Part print with two shaded views. Sizes in mm from the minimum x, y, z corner. Give positions to 0.01 mm unless a question says otherwise; leave off trailing zeros. Write each loop counter-clockwise with the first axis right and the second up, starting at its lowest first coordinate (ties: lowest second). Pieces come first, ordered by that corner, then holes. Notation, with made-up numbers: (59, -22) -> (76, -22) arc R26 cw to (76, 6) -> close; hole circle Ø9 at (83, -26). An arc over 180 degrees is marked (long way). Answer as a JSON object with one key per item and string values.
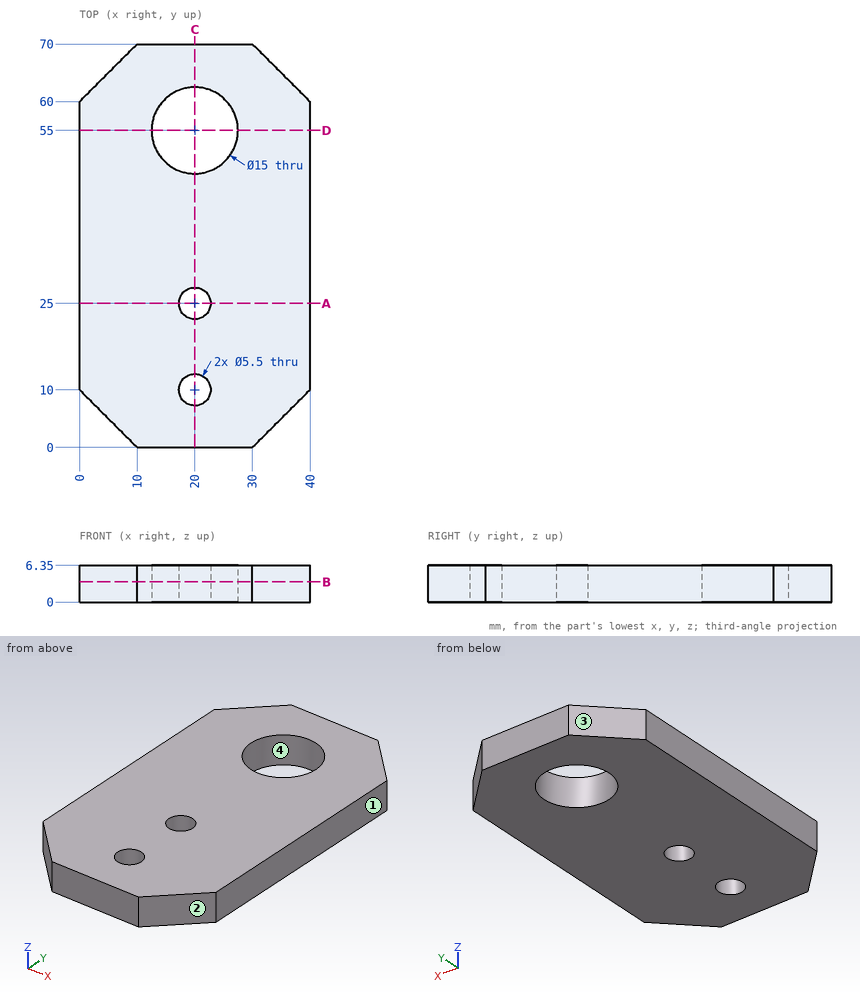
1) Mould opens along Y. For the marked faces 1, 2, 3 and 4 say: released by +Y, released by -Y, zero draft, split by the parting line, or undercut.
Model answer:
{"face 1": "zero draft", "face 2": "released by -Y", "face 3": "released by +Y", "face 4": "undercut"}
2) Slice it at B-B (z = 3.5). List the corners of the cut face in (x, y), then the cut area to 3 significant figures.
Model answer:
{"outline": "(0, 10) -> (10, 0) -> (30, 0) -> (40, 10) -> (40, 60) -> (30, 70) -> (10, 70) -> (0, 60) -> close; hole circle Ø15 at (20, 55); hole circle Ø5.5 at (20, 10); hole circle Ø5.5 at (20, 25)", "area": "2,380 mm2"}
3) Slice it at C-C (x = 20). List the corners of the cut face in (y, z).
Model answer:
{"outline": "(0, 0) -> (7.25, 0) -> (7.25, 6.35) -> (0, 6.35) -> close; (12.75, 0) -> (22.25, 0) -> (22.25, 6.35) -> (12.75, 6.35) -> close; (27.75, 0) -> (47.5, 0) -> (47.5, 6.35) -> (27.75, 6.35) -> close; (62.5, 0) -> (70, 0) -> (70, 6.35) -> (62.5, 6.35) -> close"}
4) Slice it at D-D (y = 55). List the corners of the cut face in (x, z).
Model answer:
{"outline": "(0, 0) -> (12.5, 0) -> (12.5, 6.35) -> (0, 6.35) -> close; (27.5, 0) -> (40, 0) -> (40, 6.35) -> (27.5, 6.35) -> close"}
5) Slice it at A-A (y = 25). List the corners of the cut face in (x, z), then the cut area to 3 significant figures.
Model answer:
{"outline": "(0, 0) -> (17.25, 0) -> (17.25, 6.35) -> (0, 6.35) -> close; (22.75, 0) -> (40, 0) -> (40, 6.35) -> (22.75, 6.35) -> close", "area": "219 mm2"}
6) Wall check: probe 1 along Y at (x, z) = (20, 4.25); probe 2 along Y at (x, z) = (19, 5.25); probe 3 along Y at (x, z) = (13.5, 5.5). Give the ranges that are in metal, low to high.
Model answer:
{"probe 1": "y = 0 to 7.25, 12.75 to 22.25, 27.75 to 47.5, 62.5 to 70", "probe 2": "y = 0 to 7.44, 12.56 to 22.44, 27.56 to 47.57, 62.43 to 70", "probe 3": "y = 0 to 51.26, 58.74 to 70"}
